Answer from the drawing. Dimensions are ordinates in mm from the lowest x, y and z of the part. A direction names the side the tool comes from. Give positions to 0.01 mm unless a question says otherwise; leave off trailing zeros. Order: outer loops, then holes, each group sorted by start corner. A loop starts at its lowest first (then second) coordinate and runs counter-clockwise, first axis right, second up. Notation, with made-up numbers: (43.25, -12) - (59.25, -12) arc R26 cw to (59.25, 10) - close; hole circle Ø6 at (68.25, 53). An arc over 180 degrees is marked (long way). Write each question's results on one line, items separated by ' | '.
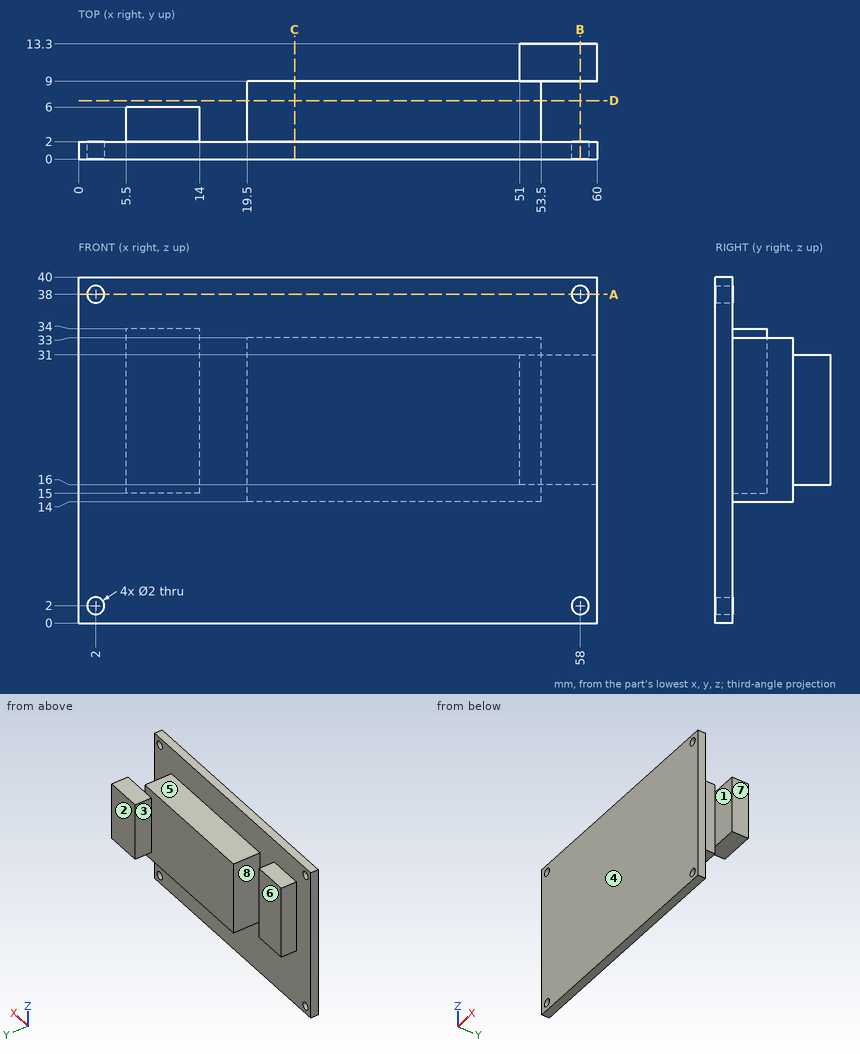
(1) Section A-A (z = 38) is taken. Give the vertices of the cut face in (x, y), plus the area to 3 significant figures.
Conclusion:
outline: (0, 0) - (1, 0) - (1, 2) - (0, 2) - close; (3, 0) - (57, 0) - (57, 2) - (3, 2) - close; (59, 0) - (60, 0) - (60, 2) - (59, 2) - close | area: 112 mm^2
(2) For the marked faces 5, 6, 7 and 8, determine the directions among +Z, -Z, +X, -X, +Y, -Y from which every point of the face is accessible in a straight line to the end or side of a thin tool.
Conclusion:
face 5: +Z, +X, +Y | face 6: +Z, -Z, -X, +Y | face 7: +Z, -Z, +X, +Y, -Y | face 8: +Z, -Z, +Y
(3) Section C-C (x = 25) is taken. Give the vertices of the cut face in (y, z), plus the area to 3 significant figures.
Conclusion:
outline: (0, 0) - (2, 0) - (2, 14) - (9, 14) - (9, 33) - (2, 33) - (2, 40) - (0, 40) - close | area: 213 mm^2
(4) Each of these flat-tipped pins is pushed along its axis until it touches: pin 1 (2 mm diameter, centred on x = 39.5, y = 6, fed in from +Z); pin 2 (5 mm diameter, centred on x = 58.5, z = 25.5, fed in from -Y); pin 3 (2 mm diameter, centred on x = 9.5, y = 4, fed in from +Z); pin 4 (3 mm diameter, centred on x = 29, y = 5, fed in from -Z). Where does it stop, or does it pass through?
Conclusion:
pin 1: z = 33 | pin 2: y = 0 | pin 3: z = 34 | pin 4: z = 14
(5) Consider probe 1 along X at (y, z) = (0.85, 38); probe 2 along Z at (x, y) = (2, 0.4); probe 3 along Y at (x, z) = (38.5, 10). Determine where each line is inside the solid, lowest interval first. Write a range as [from, to].
Conclusion:
probe 1: [0, 1], [3, 57], [59, 60] | probe 2: [0, 1], [3, 37], [39, 40] | probe 3: [0, 2]
(6) Section D-D (y = 6.75) is taken. Give the vertices of the cut face in (x, z), plus the area to 3 significant figures.
Conclusion:
outline: (19.5, 14) - (53.5, 14) - (53.5, 33) - (19.5, 33) - close | area: 646 mm^2
(7) The mould has two halves that part along Y. Classify the marked faces 1, 2, 3 and 4: pulls with the +Y half, pulls with the -Y half, needs draft (parallel to the pull), parting line crosses it, or undercut.
Conclusion:
face 1: undercut | face 2: pulls with the +Y half | face 3: needs draft | face 4: pulls with the -Y half
(8) Section B-B (x = 58) is taken. Give the vertices of the cut face in (y, z).
Conclusion:
outline: (0, 0) - (2, 0) - (2, 1) - (0, 1) - close; (0, 3) - (2, 3) - (2, 37) - (0, 37) - close; (0, 39) - (2, 39) - (2, 40) - (0, 40) - close; (9, 16) - (13.3, 16) - (13.3, 31) - (9, 31) - close
